from build123d import *

# Parameters (mm, degrees)
EXTRUDE_1_DEPTH          = 20
SKETCH_3_W               = 10
SKETCH_3_H               = 30
EXTRUDE_2_DEPTH          = 30
SKETCH_5_W               = 40
SKETCH_5_H               = 20
EXTRUDE_3_DEPTH          = 42
SKETCH_2_R               = 5
CUT_EXTRUDE_1_DEPTH      = 13
CUT_EXTRUDE_2_REACH      = 17
SKETCH_4_R               = 5
CUT_EXTRUDE_3_REACH      = 44
SKETCH_6_R               = 5
SKETCH_7_R               = 9
SKETCH_7_R_2             = 5
EXTRUDE_4_DEPTH          = 2
SKETCH_8_R               = 9
SKETCH_8_R_2             = 5
EXTRUDE_5_DEPTH          = 2
SKETCH_9_R               = 9
SKETCH_9_R_2             = 5
EXTRUDE_6_DEPTH          = 2
SKETCH_10_R              = 4
CUT_EXTRUDE_4_DEPTH      = 21
SKETCH_11_W              = 40
SKETCH_11_H              = 16
EXTRUDE_7_DEPTH          = 57
SKETCH_12_W              = 20
SKETCH_12_H              = 16
REVOLVE_1_ANGLE          = 180
SKETCH_13_R              = 15
CUT_EXTRUDE_5_DEPTH      = 35
CUT_EXTRUDE_5_DEPTH_BACK = 3
CUT_EXTRUDE_6_REACH      = 139
SKETCH_14_R              = 13
SKETCH_15_R              = 3
CUT_EXTRUDE_7_DEPTH      = 12
SKETCH_16_W              = 9.5
SKETCH_16_H              = 10
SKETCH_17_W              = 21
SKETCH_17_H              = 20
CUT_EXTRUDE_8_DEPTH      = 12
SKETCH_18_R              = 3
CUT_EXTRUDE_9_DEPTH      = 40
SKETCH_19_R              = 3
CUT_EXTRUDE_10_DEPTH     = 40
SKETCH_20_W              = 30
SKETCH_20_H              = 20
EXTRUDE_8_DEPTH          = 32
CUT_EXTRUDE_11_REACH     = 60
SKETCH_21_R              = 5


with BuildPart() as part:
    # 草图1 → 凸台-拉伸1 (new body)
    with BuildSketch(Plane(origin=(0, 0, 0), x_dir=(1, 0, 0), z_dir=(0, 1, 0))):
        Polygon((-102, 136), (-41.5, 136), (-41.5, 174), (41.5, 174), (41.5, 136), (102, 136), (102, 106), (126.5, 106), (126.5, 52), (107, 52), (107, 22), (67, 22), (67, 0), (-67, 0), (-67, 22), (-107, 22), (-107, 52), (-148.5, 52), (-148.5, 106), (-102, 106), align=None)
    extrude(amount=EXTRUDE_1_DEPTH)

    # 草图3 → 凸台-拉伸2 (add)
    with BuildSketch(Plane(origin=(0, 20, 0), x_dir=(1, 0, 0), z_dir=(0, 1, 0))):
        with Locations((-138.5, 77)):
            Rectangle(SKETCH_3_W, SKETCH_3_H)
    extrude(amount=EXTRUDE_2_DEPTH)

    # 草图5 → 凸台-拉伸3 (add)
    with BuildSketch(Plane(origin=(0, 20, 0), x_dir=(1, 0, 0), z_dir=(0, 1, 0))):
        with Locations((-87, 32)):
            Rectangle(SKETCH_5_W, SKETCH_5_H)
        with Locations((87, 32)):
            Rectangle(SKETCH_5_W, SKETCH_5_H)
    extrude(amount=EXTRUDE_3_DEPTH)

    # 草图2 → 切除-拉伸1 (cut)
    with BuildSketch(Plane(origin=(0, 20, 0), x_dir=(1, 0, 0), z_dir=(0, 1, 0))):
        with Locations((0, 103)):
            Circle(SKETCH_2_R)
        with Locations((-41, 56)):
            Circle(SKETCH_2_R)
        with Locations((41, 56)):
            Circle(SKETCH_2_R)
    extrude(amount=-CUT_EXTRUDE_1_DEPTH, mode=Mode.SUBTRACT)

    # 草图4 → 切除-拉伸2 (cut, up to next)
    with BuildSketch(Plane(origin=(-133.5, 0, 0), x_dir=(0, 0, -1), z_dir=(1, 0, 0)), mode=Mode.PRIVATE) as cut_extrude_2_sk1:
        with Locations((77, 38)):
            Circle(SKETCH_4_R)
    cut_extrude_2_tool1 = extrude(cut_extrude_2_sk1.sketch, amount=-CUT_EXTRUDE_2_REACH, mode=Mode.PRIVATE) & part.part
    add(cut_extrude_2_tool1.solids().sort_by_distance((-133.5, 38, -77))[0], mode=Mode.SUBTRACT)

    # 草图6 → 切除-拉伸3 (cut, up to next)
    with BuildSketch(Plane(origin=(0, 0, -42), x_dir=(-1, 0, 0), z_dir=(0, 0, -1)), mode=Mode.PRIVATE) as cut_extrude_3_sk1:
        with Locations((87, 38)):
            Circle(SKETCH_6_R)
    cut_extrude_3_tool1 = extrude(cut_extrude_3_sk1.sketch, amount=-CUT_EXTRUDE_3_REACH, mode=Mode.PRIVATE) & part.part
    add(cut_extrude_3_tool1.solids().sort_by_distance((-87, 38, -42))[0], mode=Mode.SUBTRACT)
    # 草图6 → 切除-拉伸3 (cut, up to next)
    with BuildSketch(Plane(origin=(0, 0, -42), x_dir=(-1, 0, 0), z_dir=(0, 0, -1)), mode=Mode.PRIVATE) as cut_extrude_3_sk2:
        with Locations((-87, 38)):
            Circle(SKETCH_6_R)
    cut_extrude_3_tool2 = extrude(cut_extrude_3_sk2.sketch, amount=-CUT_EXTRUDE_3_REACH, mode=Mode.PRIVATE) & part.part
    add(cut_extrude_3_tool2.solids().sort_by_distance((87, 38, -42))[0], mode=Mode.SUBTRACT)

    # 草图7 → 凸台-拉伸4 (add)
    with BuildSketch(Plane(origin=(-133.5, 0, 0), x_dir=(0, 0, -1), z_dir=(1, 0, 0))):
        with Locations((77, 38)):
            Circle(SKETCH_7_R)
        with Locations((77, 38)):
            Circle(SKETCH_7_R_2, mode=Mode.SUBTRACT)
    extrude(amount=EXTRUDE_4_DEPTH)

    # 草图8 → 凸台-拉伸5 (add)
    with BuildSketch(Plane(origin=(0, 0, -42), x_dir=(-1, 0, 0), z_dir=(0, 0, -1))):
        with Locations((-87, 38)):
            Circle(SKETCH_8_R)
        with Locations((-87, 38)):
            Circle(SKETCH_8_R_2, mode=Mode.SUBTRACT)
        with Locations((87, 38)):
            Circle(SKETCH_8_R)
        with Locations((87, 38)):
            Circle(SKETCH_8_R_2, mode=Mode.SUBTRACT)
    extrude(amount=EXTRUDE_5_DEPTH)

    # 草图9 → 凸台-拉伸6 (add)
    with BuildSketch(Plane(origin=(0, 20, 0), x_dir=(1, 0, 0), z_dir=(0, 1, 0))):
        with Locations((-41, 56)):
            Circle(SKETCH_9_R)
        with Locations((-41, 56)):
            Circle(SKETCH_9_R_2, mode=Mode.SUBTRACT)
        with Locations((0, 103)):
            Circle(SKETCH_9_R)
        with Locations((0, 103)):
            Circle(SKETCH_9_R_2, mode=Mode.SUBTRACT)
        with Locations((41, 56)):
            Circle(SKETCH_9_R)
        with Locations((41, 56)):
            Circle(SKETCH_9_R_2, mode=Mode.SUBTRACT)
    extrude(amount=EXTRUDE_6_DEPTH)

    # 草图10 → 切除-拉伸4 (cut, through all)
    with BuildSketch(Plane(origin=(0, 20, 0), x_dir=(1, 0, 0), z_dir=(0, 1, 0))):
        with Locations((-41, 35.75)):
            Circle(SKETCH_10_R)
        with Locations((41, 35.75)):
            Circle(SKETCH_10_R)
        with Locations((-41, 13.75)):
            Circle(SKETCH_10_R)
        with Locations((41, 13.75)):
            Circle(SKETCH_10_R)
        with Locations((-91, 79)):
            Circle(SKETCH_10_R)
        with Locations((0, 123.25)):
            Circle(SKETCH_10_R)
        with Locations((0, 145.25)):
            Circle(SKETCH_10_R)
        with Locations((85.5, 79)):
            Circle(SKETCH_10_R)
    extrude(amount=-CUT_EXTRUDE_4_DEPTH, mode=Mode.SUBTRACT)

    # 草图11 → 凸台-拉伸7 (add)
    with BuildSketch(Plane(origin=(0, 20, 0), x_dir=(1, 0, 0), z_dir=(0, 1, 0))):
        with Locations((0, 42)):
            Rectangle(SKETCH_11_W, SKETCH_11_H)
    extrude(amount=EXTRUDE_7_DEPTH)

    # 草图12 → 旋转1 (revolve)
    with BuildSketch(Plane(origin=(0, 77, 0), x_dir=(1, 0, 0), z_dir=(0, 1, 0))):
        with Locations((-10, 42)):
            Rectangle(SKETCH_12_W, SKETCH_12_H)
    revolve(axis=Axis((0, 77, -50), (0, 0, -1)), revolution_arc=REVOLVE_1_ANGLE)

    # 草图13 → 切除-拉伸5 (cut, two sides)
    with BuildSketch(Plane.XY.offset(-34)) as cut_extrude_5_sk:
        with Locations((0, 77)):
            Circle(SKETCH_13_R)
    extrude(amount=CUT_EXTRUDE_5_DEPTH, mode=Mode.SUBTRACT)
    extrude(cut_extrude_5_sk.sketch, amount=-CUT_EXTRUDE_5_DEPTH_BACK, mode=Mode.SUBTRACT)

    # 草图14 → 切除-拉伸6 (cut, up to next)
    with BuildSketch(Plane.XY.offset(-37), mode=Mode.PRIVATE) as cut_extrude_6_sk1:
        with Locations((0, 77)):
            Circle(SKETCH_14_R)
    cut_extrude_6_tool1 = extrude(cut_extrude_6_sk1.sketch, amount=-CUT_EXTRUDE_6_REACH, mode=Mode.PRIVATE) & part.part
    add(cut_extrude_6_tool1.solids().sort_by_distance((0, 77, -37))[0], mode=Mode.SUBTRACT)

    # 草图15 → 切除-拉伸7 (cut)
    with BuildSketch(Plane.XY.offset(-34)):
        with Locations((0, 57)):
            Circle(SKETCH_15_R)
    extrude(amount=-CUT_EXTRUDE_7_DEPTH, mode=Mode.SUBTRACT)

    # 草图16 → 旋转2 (revolve)
    with BuildSketch(Plane(origin=(0, 62, 0), x_dir=(1, 0, 0), z_dir=(0, 1, 0))):
        with Locations((-102.25, 37)):
            Rectangle(SKETCH_16_W, SKETCH_16_H)
        with Locations((-71.75, 37)):
            Rectangle(SKETCH_16_W, SKETCH_16_H)
        with Locations((102.25, 37)):
            Rectangle(SKETCH_16_W, SKETCH_16_H)
        with Locations((71.75, 37)):
            Rectangle(SKETCH_16_W, SKETCH_16_H)
    revolve(axis=Axis((107, 62, -32), (-1, 0, 0)))

    # 草图17 → 切除-拉伸8 (cut)
    with BuildSketch(Plane(origin=(0, 62, 0), x_dir=(1, 0, 0), z_dir=(0, 1, 0))):
        with Locations((-87, 32)):
            Rectangle(SKETCH_17_W, SKETCH_17_H)
        with Locations((87, 32)):
            Rectangle(SKETCH_17_W, SKETCH_17_H)
    extrude(amount=-CUT_EXTRUDE_8_DEPTH, mode=Mode.SUBTRACT)

    # 草图18 → 切除-拉伸9 (cut)
    with BuildSketch(Plane.ZY.offset(107)):
        with Locations((-32, 62)):
            Circle(SKETCH_18_R)
    extrude(amount=-CUT_EXTRUDE_9_DEPTH, mode=Mode.SUBTRACT)

    # 草图19 → 切除-拉伸10 (cut)
    with BuildSketch(Plane(origin=(107, 0, 0), x_dir=(0, 0, -1), z_dir=(1, 0, 0))):
        with Locations((32, 62)):
            Circle(SKETCH_19_R)
    extrude(amount=-CUT_EXTRUDE_10_DEPTH, mode=Mode.SUBTRACT)

    # 草图20 → 凸台-拉伸8 (add)
    with BuildSketch(Plane(origin=(0, 20, 0), x_dir=(1, 0, 0), z_dir=(0, 1, 0))):
        with Locations((-87, 126)):
            Rectangle(SKETCH_20_W, SKETCH_20_H)
        with Locations((87, 126)):
            Rectangle(SKETCH_20_W, SKETCH_20_H)
    extrude(amount=EXTRUDE_8_DEPTH)

    # 草图21 → 切除-拉伸11 (cut, up to next)
    with BuildSketch(Plane.XY.offset(-116), mode=Mode.PRIVATE) as cut_extrude_11_sk1:
        with Locations((87, 38)):
            Circle(SKETCH_21_R)
    cut_extrude_11_tool1 = extrude(cut_extrude_11_sk1.sketch, amount=-CUT_EXTRUDE_11_REACH, mode=Mode.PRIVATE) & part.part
    add(cut_extrude_11_tool1.solids().sort_by_distance((87, 38, -116))[0], mode=Mode.SUBTRACT)
    # 草图21 → 切除-拉伸11 (cut, up to next)
    with BuildSketch(Plane.XY.offset(-116), mode=Mode.PRIVATE) as cut_extrude_11_sk2:
        with Locations((-87, 38)):
            Circle(SKETCH_21_R)
    cut_extrude_11_tool2 = extrude(cut_extrude_11_sk2.sketch, amount=-CUT_EXTRUDE_11_REACH, mode=Mode.PRIVATE) & part.part
    add(cut_extrude_11_tool2.solids().sort_by_distance((-87, 38, -116))[0], mode=Mode.SUBTRACT)


solid = part.part
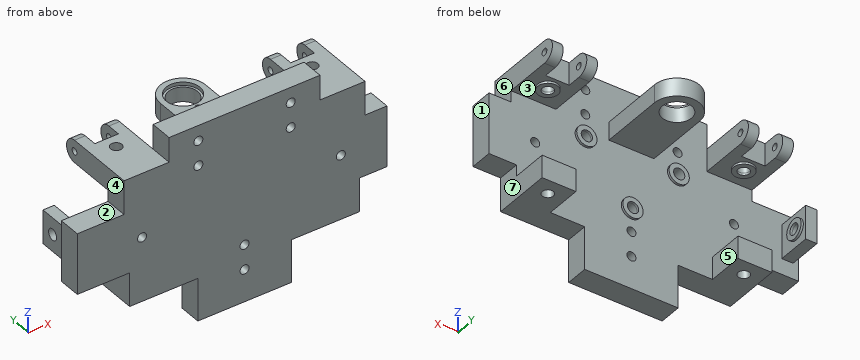
Input: part model. Units: mm. Frame: model coordinates. Face numbers are marked on the shaded views. A direction names the side the tool comes from. Give positions to 0.01 mm unless a question says otherwise; leave off trailing zeros. Order: outer loops, then holes, each group sorted by start corner. A loop starts at its lowest first (then second) coordinate and runs counter-clockwise, first axis right, second up.
Q1. Set-up query: the marked faces 4, 5, 6 and 7. Return all of +Z, -Z, +X, -X, +Y, -Y with unobstructed straight access to the full face (end or side cutting, diameter ignored); none if empty.
Checked values:
face 4: +Z, -X, +Y, -Y
face 5: -Z, +Y
face 6: +Z, +X, +Y, -Y
face 7: -Z, +X, +Y, -Y
Q2. Ray query, probe 1 along X at (y, z) = (13.5, -56); probe 2 along Z at (x, y) = (0, 12); probe 3 along Y at (x, z) = (87, -43). Return the intervals inside material, ascending.
Checked values:
probe 1: x = -148.5 to -46, -36 to 36, 46 to 126.5
probe 2: z = -174 to -149.25, -141.25 to -127.25, -119.25 to -108, -98 to 0
probe 3: y = 0 to 20, 29 to 33, 43 to 47
Q3. Draft query along Z for the marked faces 1, 2 and 3. Return one class per face: +Z half, -Z half, draft (parallel to the pull), parting line (faces both ways), or undercut.
Checked values:
face 1: draft
face 2: +Z half
face 3: undercut
Q4. Section A-A on z = -123.25. Output: boundary loops of the cut face in (x, y), and give its area (3 significant figures).
Checked values:
outline: (-102, 0) - (-4, 0) - (-4, 20) - (-72, 20) - (-72, 52) - (-102, 52) - close; (4, 0) - (102, 0) - (102, 52) - (72, 52) - (72, 20) - (4, 20) - close; hole circle Ø10 at (-87, 38); hole circle Ø10 at (87, 38)
area: 5,680 mm2
Q5. Contact query for flat-ended pins moving along their axis: pin 1 Ø8 at (x, z) = (-77, -133.5) entering from +Y; pin 2 Ø9 at (x, z) = (41.5, -58) entering from +Y; pin 3 Ø11 at (x, y) = (-138.5, 35) entering from +Z. Output: stop coordinate, or through.
Checked values:
pin 1: stops at y = 52
pin 2: stops at y = 22
pin 3: stops at z = -62
Q6. Section D-D on x = 0. State how many separate pieces and enclosed holes the cut face has, and give its area (3 significant figures).
Checked values:
separate pieces: 4
enclosed holes: 0
area: 3,780 mm2
Q7. Section B-B on y = 25.5. Output: boundary loops of the cut face in (x, z), and give its area (3 significant figures).
Checked values:
outline: (-143.5, -92) - (-133.5, -92) - (-133.5, -62) - (-143.5, -62) - close; (-107, -42) - (-67, -42) - (-67, -22) - (-107, -22) - close; (-102, -136) - (-72, -136) - (-72, -116) - (-102, -116) - close; (-20, -50) - (20, -50) - (20, -34) - (-20, -34) - close; (67, -42) - (107, -42) - (107, -22) - (67, -22) - close; (72, -136) - (102, -136) - (102, -116) - (72, -116) - close
area: 3,740 mm2
Q8. Section C-C on z = -79. Output: boundary loops of the cut face in (x, y), and give its area (3 significant figures).
Checked values:
outline: (-148.5, 0) - (-95, 0) - (-95, 20) - (-133.5, 20) - (-133.5, 29.23) - (-131.5, 29.23) - (-131.5, 33.42) - (-143.5, 33.42) - (-143.5, 20) - (-148.5, 20) - close; (-143.5, 42.58) - (-131.5, 42.58) - (-131.5, 46.77) - (-133.5, 46.77) - (-133.5, 50) - (-143.5, 50) - close; (-87, 0) - (81.5, 0) - (81.5, 20) - (-87, 20) - close; (89.5, 0) - (126.5, 0) - (126.5, 20) - (89.5, 20) - close
area: 5,410 mm2
